Autodesk Inventor part; units mm, degrees
ref_plane "YZ Plane" through (0, 0, 0) normal (1, 0, 0) x (0, 1, 0)
ref_plane "XZ Plane" through (0, 0, 0) normal (0, 1, 0) x (-1, 0, 0)
ref_plane "XY Plane" through (0, 0, 0) normal (0, 0, 1) x (1, 0, 0)
sketch "Boceto1" plane through (0, 0, 0) normal (0, 0, 1) x (1, 0, 0)
  line L0 (-4.25, 9.25) -> (4.25, 9.25)
  line L1 (9.25, 4.25) -> (9.25, -4.25)
  line L2 (4.25, -9.25) -> (-4.25, -9.25)
  line L3 (-9.25, -4.25) -> (-9.25, 4.25)
  arc A0 (-4.25, 9.25) -> (-9.25, 4.25) centre (-4.25, 4.25) ccw
  arc A1 (-9.25, -4.25) -> (-4.25, -9.25) centre (-4.25, -4.25) ccw
  arc A2 (4.25, -9.25) -> (9.25, -4.25) centre (4.25, -4.25) ccw
  arc A3 (9.25, 4.25) -> (4.25, 9.25) centre (4.25, 4.25) ccw
  line L4 (-3.25, 3.25) -> (3.25, 3.25)
  line L5 (3.25, 3.25) -> (3.25, -3.25)
  line L6 (3.25, -3.25) -> (-3.25, -3.25)
  line L7 (-3.25, -3.25) -> (-3.25, 3.25)
  line L8 (-3.25, 3.25) -> (3.25, -3.25) construction
  line L9 (3.25, 3.25) -> (-3.25, -3.25) construction
  point P0 (0, 0)
  dimension "d32" = 6.5
  dimension "d33" = 6.5
extrude "Extrusión1" add sketch "Boceto1" against normal blind 2.5
sketch "Boceto3" plane through (0, 0, -2.5) normal (0, 0, -1) x (-1, 0, 0)
  line L0 (-5, -5) -> (5, -5)
  line L1 (5, -5) -> (5, 5)
  line L2 (5, 5) -> (-5, 5)
  line L3 (-5, 5) -> (-5, -5)
  line L4 (-3.25, 3.25) -> (3.25, 3.25)
  line L5 (3.25, 3.25) -> (3.25, -3.25)
  line L6 (3.25, -3.25) -> (-3.25, -3.25)
  line L7 (-3.25, -3.25) -> (-3.25, 3.25)
extrude "Extrusión2" add sketch "Boceto3" along normal blind 25
sketch "Boceto4" plane through (0, 0, 0) normal (0, 0, 1) x (1, 0, 0)
  line L0 (-3.65, 8.15) -> (3.65, 8.15)
  line L1 (8.15, 3.65) -> (8.15, -3.65)
  line L2 (3.65, -8.15) -> (-3.65, -8.15)
  line L3 (-8.15, -3.65) -> (-8.15, 3.65)
  arc A0 (3.65, -8.15) -> (8.15, -3.65) centre (3.65, -3.65) ccw
  arc A1 (-8.15, -3.65) -> (-3.65, -8.15) centre (-3.65, -3.65) ccw
  arc A2 (-3.65, 8.15) -> (-8.15, 3.65) centre (-3.65, 3.65) ccw
  arc A3 (8.15, 3.65) -> (3.65, 8.15) centre (3.65, 3.65) ccw
  line L4 (-2.5, 6) -> (2.5, 6)
  line L5 (6, 2.5) -> (6, -2.5)
  line L6 (2.5, -6) -> (-2.5, -6)
  line L7 (-6, -2.5) -> (-6, 2.5)
  arc A4 (6, 2.5) -> (2.5, 6) centre (2.5, 2.5) ccw
  arc A5 (2.5, -6) -> (6, -2.5) centre (2.5, -2.5) ccw
  arc A6 (-6, -2.5) -> (-2.5, -6) centre (-2.5, -2.5) ccw
  arc A7 (-2.5, 6) -> (-6, 2.5) centre (-2.5, 2.5) ccw
extrude "Extrusión3" add sketch "Boceto4" along normal blind 9.5
properties part number "_3DPrint"
Here's how the part is built. I have some questions about the finished solid (model axes, mm). A direction names the side the tool comes from. Give positions to 0.01 mm unless a question says otherwise; leave off trailing zeros. Order: outer loops, then holes, each group sorted by start corner. A loop starts at its lowest first (then second) coordinate and runs counter-clockwise, first axis right, second up. Notation, with made-up numbers: (77.5, 55.5) - (134.5, 55.5) arc R24 cw to (134.5, 81.5) - close; hole circle Ø11 at (-7.75, -11.5). An arc over 180 degrees is marked (long way). Answer as a JSON object with one key per item and string values. Group by question number.
Item 1: Which directions (+Z, -Z, +X, -X, +Y, -Y) give clear straight access to the entire face, cutting with the end or side of a thin tool? Please do faces 5 (the cylindrical face through (6.797, 6.867, 4.684)), 6 (the flat face through (-4, 0, 0)), 7 (the flat face through (0, -5, -15)), 8 (the flat face through (8.15, 0, 5)), 9 (the flat face through (0, -8.15, 5)).
Item 2: If we section it at B-B on x = 0.75: Please give me the cut outline in (y, z), and give its area (3 significant figures).
Item 3: For P1, Ø6, axis at x = 1.5, y = 2, coming from the +Z side; P2, Ø5, axis at x = -0.5, z = -14, coming from the -Y side; P3, Ø7, axis at y = 0.5, z = -17.5, coming from the +X side, each with a flat end and sliding along its axis, tell me the tip position at first contact or that it passes through.
Item 4: If we mould it in two halves opening along X, with no side actions, what happens to faces 1 (the cylindrical face through (4.95, 5, 4.68)), 2 (the flat face through (6, 0, 5)), 3 (the cylindrical face through (6.867, -6.797, 4.684)), 4 (the flat face through (-8.3, 0, 0))? For each: pulls with the +X half, pulls with the -X half, needs draft (parallel to the pull), parting line crosses it, or undercut.
Item 5: Please list where these lines run through material, in increasing order: probe 1 along Y at (x, z) = (0.5, -4.5); probe 2 along Y at (x, z) = (-1.75, 0.5).
Item 6: If we section it at D-D on z = -11: Please give me the cut outline in (x, y), and give its area (4 significant figures).
Item 7: If we section it at A-A on z = 6.5: Please give me the cut outline in (x, y).
Item 8: If we section it at C-C on y = 5.5: Please give me the cut outline in (x, z).
Result set:
{
 "1": {"face 5": "+Z, +X, +Y", "face 6": "+Z", "face 7": "-Z, +X, -X, -Y", "face 8": "+Z, +X, +Y, -Y", "face 9": "+Z, +X, -X, -Y"},
 "2": {"outline": "(-9.25, -2.5) - (-5, -2.5) - (-5, -27.5) - (-3.25, -27.5) - (-3.25, 0) - (-6, 0) - (-6, 9.5) - (-8.15, 9.5) - (-8.15, 0) - (-9.25, 0) - close; (3.25, -27.5) - (5, -27.5) - (5, -2.5) - (9.25, -2.5) - (9.25, 0) - (8.15, 0) - (8.15, 9.5) - (6, 9.5) - (6, 0) - (3.25, 0) - close", "area": "158 mm²"},
 "3": {"P1": "z = 0", "P2": "y = -5", "P3": "x = 5"},
 "4": {"face 1": "undercut", "face 2": "undercut", "face 3": "pulls with the +X half", "face 4": "needs draft"},
 "5": {"probe 1": "-5 to -3.25, 3.25 to 5", "probe 2": "-8.15 to -6, 6 to 8.15"},
 "6": {"outline": "(-5, -5) - (5, -5) - (5, 5) - (-5, 5) - close; hole (-3.25, -3.25) - (3.25, -3.25) - (3.25, 3.25) - (-3.25, 3.25) - close", "area": "57.75 mm²"},
 "7": {"outline": "(-8.15, -3.65) arc R4.5 ccw to (-3.65, -8.15) - (3.65, -8.15) arc R4.5 ccw to (8.15, -3.65) - (8.15, 3.65) arc R4.5 ccw to (3.65, 8.15) - (-3.65, 8.15) arc R4.5 ccw to (-8.15, 3.65) - close; hole (-6, -2.5) arc R3.5 ccw to (-2.5, -6) - (2.5, -6) arc R3.5 ccw to (6, -2.5) - (6, 2.5) arc R3.5 ccw to (2.5, 6) - (-2.5, 6) arc R3.5 ccw to (-6, 2.5) - close"},
 "8": {"outline": "(-9.09, -2.5) - (9.09, -2.5) - (9.09, 0) - (7.75, 0) - (7.75, 9.5) - (4.3, 9.5) - (4.3, 0) - (-4.3, 0) - (-4.3, 9.5) - (-7.75, 9.5) - (-7.75, 0) - (-9.09, 0) - close"}
}
